Input: part model. Units: mm. Frame: model coordinates. A direction names the side the tool comes from. Coordinates: 2 decimals unless noted, no trailing zeros. Loops run counter-clockwise (first coordinate to the right, second up) from the corner with the lowest first, then second, coordinate; pieces in that order, holes last.
Item 1: Reachability of faces 1 (the flat face through (82, -25, -38.1)), 2 (the flat face through (81, -25, 0)), 3 (the flat face through (-80, -25, 0)) from +Z, -Z, +X, -X, +Y, -Y: full face, straight path, thin tool, end or side. Return the list, or none.
Item 2: Section D-D on z = -34. Return loops of the section in (x, y), and give its area (3 significant figures).
Item 3: Section A-A on y = -17. Return loops of the section in (x, z), and give its area (3 significant figures).
Item 4: Section C-C on x = -41.5. Return loops of the section in (y, z), and give its area (3 significant figures).
Item 5: Contact query for a flat-ended pin moving along its axis: P1, Ø5, axis at x = 27, y = -18, coming from the -Z side. Output: stop coordinate, or through.
Item 6: Ray query, line 1 along Z through (x, y) = (-117, -44); line 2 along Z through (x, y) = (-0.5, -49); line 3 along X through (y, z) = (-40.5, -9). Return the intervals inside material, ascending.
Item 7: Pull-direction query (X, two-part tool) for faces 4 (the cylindrical face through (0.514, -25.044, 12.697)), 5 (the flat face through (-83, -25, -38.1)), 6 (the cylindrical face through (-0.84, -25.04, -0.01)); classes: released by +X, released by -X, zero draft, split by the parting line, or undercut.
Item 8: Section B-B on z = -6.5. Return loops of the section in (x, y), and give its area (3 significant figures).
```python
from build123d import *

# Parameters (mm, degrees)
F1_DEPTH = 50.8


with BuildPart() as f1:
    # F0 (on Front) → F1 (new body)
    with BuildSketch(Plane.XZ):
        with BuildLine():
            Line((-127, 0), (-127, -38.1))
            Line((-127, -38.1), (-50.8, -38.1))
            ThreePointArc((-50.8, -38.1), (-46.301042, -17.198958), (-33.601042, 0))
            Line((-33.601042, 0), (-127, 0))
        make_face()
        with BuildLine():
            Line((127, 0), (33.601042, 0))
            ThreePointArc((33.601042, 0), (46.301042, -17.198958), (50.8, -38.1))
            Line((50.8, -38.1), (127, -38.1))
            Line((127, -38.1), (127, 0))
        make_face()
        with BuildLine():
            ThreePointArc((-33.601042, 0), (-46.301042, -17.198958), (-50.8, -38.1))
            Line((-50.8, -38.1), (-38.1, -38.1))
            ThreePointArc((-38.1, -38.1), (0, 0), (38.1, -38.1))
            Line((38.1, -38.1), (50.8, -38.1))
            ThreePointArc((50.8, -38.1), (46.301042, -17.198958), (33.601042, 0))
            ThreePointArc((33.601042, 0), (0, 12.7), (-33.601042, 0))
        make_face()
    extrude(amount=F1_DEPTH)


solid = f1.part
```
Results found:
1. face 1: -Z, +X, -X, +Y, -Y
1. face 2: +Z, +X, +Y, -Y
1. face 3: +Z, -X, +Y, -Y
2. outline: (-127, -50.8) - (-37.88, -50.8) - (-37.88, 0) - (-127, 0) - close; (37.88, -50.8) - (127, -50.8) - (127, 0) - (37.88, 0) - close
2. area: 9,050 mm2
3. outline: (-127, -38.1) - (-38.1, -38.1) arc R38.1 cw to (38.1, -38.1) - (127, -38.1) - (127, 0) - (33.6, 0) arc R50.8 ccw to (-33.6, 0) - (-127, 0) - close
3. area: 7,980 mm2
4. outline: (-50.8, -38.1) - (0, -38.1) - (0, 0) - (-50.8, 0) - close
4. area: 1,940 mm2
5. P1: stops at z = -13.99
6. line 1: z = -38.1 to 0
6. line 2: z = 0 to 12.7
6. line 3: x = -127 to -24.59, 24.59 to 127
7. face 4: split by the parting line
7. face 5: zero draft
7. face 6: undercut
8. outline: (-127, -50.8) - (-21.28, -50.8) - (-21.28, 0) - (-127, 0) - close; (21.28, -50.8) - (127, -50.8) - (127, 0) - (21.28, 0) - close
8. area: 10,700 mm2
